```python
from build123d import *

# Parameters (mm, degrees)
SKETCH_1_W          = 10
SKETCH_1_H          = 10
EXTRUDE_1_DEPTH     = 80
SKETCH_4_R          = 4
CUT_EXTRUDE_3_DEPTH = 75
SKETCH_5_R          = 2
CUT_EXTRUDE_4_DEPTH = 11
SKETCH_6_R          = 2
CUT_EXTRUDE_5_DEPTH = 10


with BuildPart() as part:
    # 草图1 → 凸台-拉伸1 (new body)
    with BuildSketch(Plane(origin=(0, 0, 0), x_dir=(1, 0, 0), z_dir=(0, 1, 0))):
        Rectangle(SKETCH_1_W, SKETCH_1_H)
    extrude(amount=EXTRUDE_1_DEPTH)

    # 草图4 → 切除-拉伸3 (cut)
    with BuildSketch(Plane(origin=(0, 80, 0), x_dir=(1, 0, 0), z_dir=(0, 1, 0))):
        Circle(SKETCH_4_R)
    extrude(amount=-CUT_EXTRUDE_3_DEPTH, mode=Mode.SUBTRACT)

    # 草图5 → 切除-拉伸4 (cut, through all)
    with BuildSketch(Plane(origin=(5, 0, 0), x_dir=(0, 0, -1), z_dir=(1, 0, 0))):
        with Locations((0, 65)):
            Circle(SKETCH_5_R)
    extrude(amount=-CUT_EXTRUDE_4_DEPTH, mode=Mode.SUBTRACT)

    # 草图6 → 切除-拉伸5 (cut)
    with BuildSketch(Plane(origin=(0, 0, -5), x_dir=(-1, 0, 0), z_dir=(0, 0, -1))):
        with Locations((0, 65)):
            Circle(SKETCH_6_R)
    extrude(amount=-CUT_EXTRUDE_5_DEPTH, mode=Mode.SUBTRACT)


solid = part.part
```
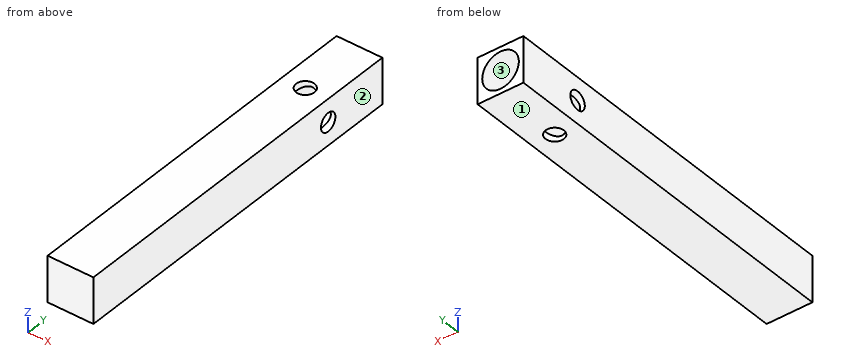
Design review of the part built by this model. Coordinates are the model's own, in mm. Face numbers are marked on the shaded views. Round coordinates to 2 decimals unless told otherwise and drop trailing zeros. Write each loop counter-clockwise with the first axis right and the second up, starting at its lowest first coordinate (ties: lowest second). Pieces come first, ordered by that corner, then holes.
Item 1: Clearance check with flat-ended pins moving along their axes: pin 1 Ø2.5 at (x, y) = (0, 65) entering from +Z; pin 2 Ø1 at (x, z) = (-1, 1.5) entering from +Y. State where each tip first meets the part, or that it passes through.
Item 2: We need section B-B on x = 0. Write out the cut boundary in (y, z), and give its area (3 significant figures).
Item 3: For probe 1 along Y at (x, z) = (0, 4.35); probe 2 along X at (y, z) = (65, -3.9); probe 3 along Z at (x, y) = (-2, 32), list the stretches that pass through material, from the lowest coordinate up.
Item 4: The part is to be moulded in two halves that separate along Z. For the marked faces 1, 2 and 3, say which applies: +Z half, -Z half, draft (parallel to the pull), parting line (faces both ways), or undercut.
Item 5: We need section C-C on y = 65. Write out the cut boundary in (x, z), and give its area (3 significant figures).
Item 6: We need section D-D on y = 48.5. Write out the cut boundary in (x, z), and give its area (3 significant figures).
Item 7: We need section A-A on z = 0. Write out the cut boundary in (x, y), and give its area (3 significant figures).
Returned:
1. pin 1: passes through
1. pin 2: stops at y = 5
2. outline: (0, -5) - (63, -5) - (63, -4) - (5, -4) - (5, 4) - (63, 4) - (63, 5) - (0, 5) - close; (67, -5) - (80, -5) - (80, -4) - (67, -4) - close; (67, 4) - (80, 4) - (80, 5) - (67, 5) - close
2. area: 192 mm2
3. probe 1: y = 0 to 63, 67 to 80
3. probe 2: x = -5 to -2, 2 to 5
3. probe 3: z = -5 to -3.46, 3.46 to 5
4. face 1: -Z half
4. face 2: draft
4. face 3: undercut
5. outline: (-5, -5) - (-2, -5) - (-2, -3.46) arc R4 cw to (-3.46, -2) - (-5, -2) - close; (-5, 2) - (-3.46, 2) arc R4 cw to (-2, 3.46) - (-2, 5) - (-5, 5) - close; (2, -5) - (5, -5) - (5, -2) - (3.46, -2) arc R4 cw to (2, -3.46) - close; (2, 3.46) arc R4 cw to (3.46, 2) - (5, 2) - (5, 5) - (2, 5) - close
5. area: 31.0 mm2
6. outline: (-5, -5) - (5, -5) - (5, 5) - (-5, 5) - close; hole circle Ø8 at (0, 0)
6. area: 49.7 mm2
7. outline: (-5, 0) - (5, 0) - (5, 63) - (4, 63) - (4, 5) - (-4, 5) - (-4, 63) - (-5, 63) - close; (-5, 67) - (-4, 67) - (-4, 80) - (-5, 80) - close; (4, 67) - (5, 67) - (5, 80) - (4, 80) - close
7. area: 192 mm2
